Design review of the part built by this model. Coordinates are the model's own, in mm. A direction names the side the tool comes from. Coordinates: 2 decimals unless noted, no trailing zeros. Loops run counter-clockwise (first coordinate to the right, second up) from the corner with the lowest first, then second, coordinate; pieces in that order, holes last. Notation, with made-up numbers: (-35, 10) - (16, 10) arc R16 ccw to (16, 36) - close; hole circle Ø8 at (-26.5, 11.5). An arc over 180 degrees is marked (long way). Use one line per item in the form item = value. Start each with the question number.
(1) Tool access review of faces 1 (the face through (81.63, 0, 0)), 2 (the face through (78.63, 1.42, -3.91)): name each direction out of +Z, -Z, +X, -X, +Y, -Y from which nothing blocks a thin tool from reaching the whole face with its end or side.
(2) Clearance check with flat-ended pins moving along their axes: pin 1 Ø1 at (x, z) = (65, 2) entering from -Y; pin 2 Ø4 at (x, y) = (19.5, -4) entering from +Z; pin 3 Ø6 at (x, z) = (55.5, 2) entering from -Y. State where each tip first meets the part, or that it passes through.
(3) For L1, parallel to X at y = -5, z = 0.5; L2, parallel to Y at x = 74.5, z = -1.75; L3, parallel to Y at x = 39.5, z = -2, list the stretches that pass through material, from the lowest coordinate up.
(4) Add section A-A (x = 24). State the section outline as (y, z) points, plus the area to 3 significant figures.
```python
from build123d import *

# Parameters (mm, degrees)
SKETCH1_R           = 4
BOSS_EXTRUDE2_DEPTH = 78.63
SKETCH2_R           = 6
BOSS_EXTRUDE3_DEPTH = 3
SKETCH3_R           = 0.2
CUT_EXTRUDE1_DEPTH  = 3
CIRPATTERN1_COUNT   = 24


with BuildPart() as part:
    # Sketch1 → Boss-Extrude2 (new body)
    with BuildSketch(Plane(origin=(0, 0, 0), x_dir=(0, 0, -1), z_dir=(1, 0, 0))):
        Circle(SKETCH1_R)
    extrude(amount=BOSS_EXTRUDE2_DEPTH)

    # Sketch2 → Boss-Extrude3 (add)
    with BuildSketch(Plane(origin=(78.63, 0, 0), x_dir=(0, 0, -1), z_dir=(1, 0, 0))):
        Circle(SKETCH2_R)
    extrude(amount=BOSS_EXTRUDE3_DEPTH)

    # Sketch3 → Cut-Extrude1 (cut)
    with BuildSketch(Plane(origin=(81.63, 0, 0), x_dir=(0, 0, -1), z_dir=(1, 0, 0))):
        with Locations((-6, 0)):
            Circle(SKETCH3_R)
    cut_extrude1 = extrude(amount=-CUT_EXTRUDE1_DEPTH, mode=Mode.SUBTRACT)

    # CirPattern1: Cut-Extrude1 ×24 about axis
    cirpattern1_axis = Axis((0, 0, -0.003264402), (1, 0, 0))
    for i in range(1, CIRPATTERN1_COUNT):
        add(cut_extrude1.rotate(cirpattern1_axis, i * 360 / CIRPATTERN1_COUNT), mode=Mode.SUBTRACT)


solid = part.part
```
Computed values:
q1.face_1 = +Z, -Z, +X, +Y, -Y
q1.face_2 = -X
q2.pin_1 = -3.71
q2.pin_2 = 3.46
q2.pin_3 = -4
q3.L1 = 78.63 to 81.63
q3.L2 = -3.6 to 3.6
q3.L3 = -3.46 to 3.46
q4.outline = circle Ø8 at (0, 0)
q4.area = 50.3 mm^2
